The listing builds one solid part. Answer for the finished solid, in the listing's coordinates (mm). A direction names the side the tool comes from. Coordinates: 2 decimals unless noted, no trailing zeros. Write each loop counter-clockwise with the first axis right and the second up, starting at its lowest first coordinate (ties: lowest second). Pieces come first, ordered by that corner, then holes.
(1) The part is cut by section B-B on y = 24.5. Determine the outline of the cut face in (x, z), plus the area to 3 significant figures.
(2) Straight lines are drawn through the part: line 1 (Z direction, x = -43, y = -25); line 2 (Z direction, x = -21.5, y = 15); line 3 (Y direction, x = -67.25, z = 25). For each, find the intervals that lie inside material, in ascending order.
(3) Which of the six approach directions +Z, -Z, +X, -X, +Y, -Y give full straight-line access (tool end or side, diameter ignored) to faces 4 (the flat face through (-11.3, -12.93, -4)), 5 (the flat face through (-60, -19, 13)), 6 (the cylindrical face through (8.716, -28.706, -0.112)), 7 (the flat face through (-10, -15, 4))?
(4) Given P1, Ø15.5, axis at y = 24.5, z = -3, coming from the +X side; P2, Ø15.5, axis at x = 26, z = 4, coming from the +Y side; P3, Ø6.5, axis at y = -16, z = 14, coming from the +X side; P4, Ø8, axis at y = 12.5, z = 13.5, coming from the -X side, each flat-ended and moving along its own axis, determine where each tip first touches the part or whether it passes through.
(5) For a pull along Z with two mould halves and no side action, classify faces 1 (the cylindrical face through (-66.4, -24.1, 19.5)), 2 (the conical face through (-11.1, -11.8, -3.2)), 3 (the flat face through (-40, -12, 5)) as +Z half, -Z half, draft (parallel to the pull), parting line (faces both ways), or undercut.
(6) The part is cut by section A-A on x = -64. Determine the outline of the cut face in (y, z), plus the area to 3 significant figures.
Autodesk Inventor part; units mm, degrees
ref_plane "YZ Plane" through (0, 0, 0) normal (1, 0, 0) x (0, 1, 0)
ref_plane "XZ Plane" through (0, 0, 0) normal (0, 1, 0) x (-1, 0, 0)
ref_plane "XY Plane" through (0, 0, 0) normal (0, 0, 1) x (1, 0, 0)
sketch "스케치1" plane through (0, 0, 0) normal (0, 0, 1) x (1, 0, 0)
  arc A0 (0, 16) -> (16, 0) centre (0, 0) ccw
  arc A1 (0, 22) -> (22, 0) centre (0, 0) ccw
  arc A2 (0, 30) -> (30, 0) centre (0, 0) ccw
  line L0 (0, -30) -> (-70, -30)
  line L1 (-70, -30) -> (-70, -8)
  line L2 (-70, -8) -> (-15.7735, 25.5185)
  line L3 (0, -30) -> (0, 30) construction
  line L4 (-30, 0) -> (30, 0) construction
  line L5 (0, 30) -> (0, 16)
  line L6 (16, 0) -> (30, 0)
  point P0 (0, 22)
  point P1 (22, 0)
  dimension "d0" = 32
  dimension "d1" = 44
  dimension "d2" = 60
  dimension "d3" = 70
  dimension "d4" = 22
extrude "돌출1" add sketch "스케치1" along normal blind 4 contours A0 L6 A1 L5
extrude "돌출2" add sketch "스케치1" along normal blind 8 contours A1 L6 A2 L5
extrude "돌출3" add sketch "스케치1" along normal blind 5 contours A2 L0 L1 L2
chamfer "모따기1" distance 1 angle 45 1 edges at (-15.5563, -15.5563, 8)
chamfer "모따기2" distance 1 angle 45 1 edges at (-11.3137, -11.3137, 4)
mirror "미러1" about plane through (0, 0, 0) normal (0, 0, -1)
ref_plane "작업 평면1" through (-70, -30, 0) normal (-1, 0, 0) x (0, 0, 1)
sketch "스케치2" plane through (-70, -30, 0) normal (-1, 0, 0) x (0, 0, 1)
  line L0 (-5, 0) -> (-5, 55.5185)
  line L1 (-5, 0) -> (25, 0)
  circle A0 centre (25, 11) radius 7.5
  circle A1 centre (25, 11) radius 11
  line L2 (25, 22) -> (-5, 22)
  line L3 (-5, 22) -> (-5, 0)
  line L4 (25, 0) -> (25, 22) construction
  point P0 (0, 30)
  dimension "d17" = 30
  dimension "d21" = 11
  dimension "d22" = 15
  dimension "d23" = 22
extrude "돌출4" add sketch "스케치2" against normal blind 10 contours L0 L2 A1 L1
extrude "돌출5" add sketch "스케치2" against normal blind 10 contours A1
extrude "돌출6" add sketch "스케치2" along normal blind 3 contours A1
chamfer "모따기3" distance 1 angle 45 1 edges at (-73, -19, 17.5)
chamfer "모따기4" distance 1 angle 45 1 edges at (-60, -19, 17.5)
properties part number "Day02_Task02"
Model answer:
1. outline: (-17.42, -5) - (-17.31, -5) - (-17.31, -8) - (0, -8) - (0, 8) - (-17.31, 8) - (-17.31, 5) - (-17.42, 5) - close
1. area: 278 mm2
2. line 1: z = -5 to 5
2. line 2: z = -8 to 8
2. line 3: y = -30 to -26.5, -11.5 to -8
3. face 4: -Z
3. face 5: +Z, +Y, -Y
3. face 6: none
3. face 7: +Z
4. P1: stops at x = 0
4. P2: stops at y = 0
4. P3: stops at x = -60
4. P4: passes through
5. face 1: undercut
5. face 2: -Z half
5. face 3: +Z half
6. outline: (-30, -5) - (-4.29, -5) - (-4.29, 5) - (-8, 5) - (-8, 25) arc R11 ccw to (-30, 25) - close; hole circle Ø15 at (-19, 25)
6. area: 710 mm2
